For this review, take the finished solid that the model builds, in its own axes (mm). Face numbers are marked on the shaded views. A direction names the side the tool comes from. Give positions to 0.01 mm unless a question says otherwise; leave off trailing zeros. Write each loop counter-clockwise with the first axis right and the second up, starting at its lowest first coordinate (ties: lowest second). Pieces come first, ordered by that corner, then holes. Notation, with made-up numbers: M 61,5.25 L 111,5.25 A34 cw 111,39.25 Z; hole C 51.25,61.5 d6. An arc over 180 degrees is marked long. Write item = value, one per line.
```python
from build123d import *

# Parameters (mm, degrees)
F0_W     = 203.2
F0_H     = 101.6
F1_DEPTH = 101.6
F3_DEPTH = 203.2
F4_W     = 101.6
F4_H     = 40.903057
F5_DEPTH = 50.8


with BuildPart() as f1:
    # F0 (on Front) → F1 (new body)
    with BuildSketch(Plane.XZ):
        with Locations((-4.904039, 9.921888)):
            Rectangle(F0_W, F0_H)
    extrude(amount=F1_DEPTH)

    # F2 (on face) → F3 (cut)
    with BuildSketch(Plane.YZ.offset(96.695961)):
        Polygon((-101.6, 60.721888), (-101.6, -15.478112), (-50.8, 60.721888), align=None)
    extrude(amount=-F3_DEPTH, mode=Mode.SUBTRACT)

    # F4 (on face) → F5 (cut)
    with BuildSketch(Plane.XY.offset(60.721888)):
        with Locations((-4.904039, -71.251529)):
            Rectangle(F4_W, F4_H)
    extrude(amount=-F5_DEPTH, mode=Mode.SUBTRACT)


solid = f1.part
```
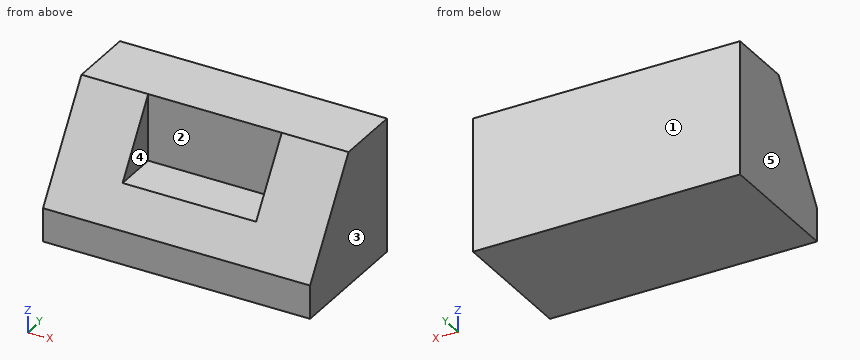
1. The part is to be moulded in two halves that separate along X. For the marked faces 1, 2 and 3, say which applies: +X half, -X half, draft (parallel to the pull), parting line (faces both ways), or undercut.
Responses:
face_1 = draft
face_2 = undercut
face_3 = +X half
2. Insertion check: P1, Ø3, axis at x = -14, z = 21.5, coming from the -Y side; P2, Ø2, axis at x = 28, z = 33, coming from the +Y side; P3, Ø4, axis at x = 52, y = -73.5, coming from the +Z side; P4, Ø2, axis at x = -63, z = 9, coming from the -Y side. Each pin has a flat end and moves straight along its axis. Give the tip position at first contact, or say it passes through.
Responses:
P1 = -50.8
P2 = 0
P3 = 29.67
P4 = -85.95
3. For line 1 along X through (y, z) = (-69.5, 22); line 2 along Y through (x, z) = (5.5, 40.5); line 3 along Z through (x, y) = (42.5, -67.5), list the stretches that pass through material, from the lowest coordinate up. Write a range as from..to.
Responses:
line_1 = -106.5..-55.7, 45.9..96.7
line_2 = -50.8..0
line_3 = -40.88..9.92
4. Machinability: for the marked faces 4 and 5, which of the approach directions +Z, -Z, +X, -X, +Y, -Y give a long, thin tool a straight path to every point of the face, cutting with its end or side? Answer none if there is none.
Responses:
face_4 = +Z, -Y
face_5 = +Z, -Z, -X, +Y, -Y
5. We need section B-B, the plane y = -78.5. Write out the cut boundary in (x, z).
Responses:
outline = M -106.5,-40.88 L 96.7,-40.88 L 96.7,19.17 L 45.9,19.17 L 45.9,9.92 L -55.7,9.92 L -55.7,19.17 L -106.5,19.17 Z
6. We need section A-A, the plane x = -23.5. Write out the cut boundary in (y, z).
Responses:
outline = M -101.6,-40.88 L 0,-40.88 L 0,60.72 L -50.8,60.72 L -50.8,9.92 L -84.67,9.92 L -101.6,-15.48 Z
7. We need section C-C, the plane z = 15. Write out the cut boundary in (x, y).
Responses:
outline = M -106.5,-81.28 L -55.7,-81.28 L -55.7,-50.8 L 45.9,-50.8 L 45.9,-81.28 L 96.7,-81.28 L 96.7,0 L -106.5,0 Z
8. We need section D-D, the plane x = 49. Write out the cut boundary in (y, z).
Responses:
outline = M -101.6,-40.88 L 0,-40.88 L 0,60.72 L -50.8,60.72 L -101.6,-15.48 Z
